Geometry: final body of the model. Coordinates: model frame, mm. Face numbers are marked on the shaded views. A direction names the side the tool comes from. Coordinates: 2 decimals unless noted, no trailing zeros. Loops run counter-clockwise (first coordinate to the right, second up) from the corner with the lowest first, then second, coordinate; pieces in that order, holes last. Notation, with made-up numbers: (-40, 10.5) -> (5, 10.5) arc R28 cw to (5, 45.5) -> close; hole circle Ø8 at (50, -9.75). An arc over 180 degrees is marked (long way). One line per item, written item: value. Start each with the question number.
Item 1: Mould query, pull axis Y, two halves, no side actions, for the marked faces 1, 2 and 3. Classes: +Y half, -Y half, draft (parallel to the pull), parting line (faces both ways), or undercut.
Item 2: Section query C-C on x = 36. Return loops of the section in (y, z) (3 decimals), then the cut area to 3 significant figures.
Item 3: Set-up query: the marked faces 4, 5, 6, 7 and 8. Return all of +Z, -Z, +X, -X, +Y, -Y with unobstructed straight access to the full face (end or side cutting, diameter ignored); none if empty.
Item 4: Section query A-A on y = 12.7. Return loops of the section in (x, z) (3 decimals), then the cut area to 3 significant figures.
Item 5: Contact query for flat-ended pins moving along their axis: pin 1 Ø4 at (x, y) = (38.5, -47.5) entering from -Z; pin 2 Ø3 at (y, z) = (-28.5, 12.5) entering from -X; pin 3 Ø3.5 at (y, z) = (-12.7, 0) entering from -X; pin 4 Ø10 at (y, z) = (-49.5, 4) entering from +X. Output: stop coordinate, or through.
Item 6: Section query B-B on y = -15. Return loops of the section in (x, z) (3 decimals), then the cut area to 3 significant figures.
Item 7: Ray query, probe 1 along X at (y, z) = (-3.5, 10); probe 2 along Y at (x, z) = (-4, 0) (3 decimals); probe 3 along Y at (x, z) = (32.1, 0) (3 decimals). Return the intervals inside material, ascending. Write a range as from..to.
Item 8: Section query D-D on x = 21.5. Return loops of the section in (y, z) (3 decimals).
from build123d import *

# Parameters (mm, degrees)
SKETCH1_R               = 15.875
SKETCH1_R_2             = 9.5
BOSS_EXTRUDE1_DEPTH     = 6
BOSS_EXTRUDE2_START     = 13.050000062
SKETCH2_R               = 15.875
SKETCH2_R_2             = 9.5
SKETCH2_R_3             = 7.62
BOSS_EXTRUDE2_DEPTH     = 13.050000062
BOSS_EXTRUDE3_START     = -19.050000062
BOSS_EXTRUDE3_DEPTH     = 19.050000062
BOSS_EXTRUDE4_START     = 21.59
BOSS_EXTRUDE4_DEPTH     = 19.050000062
BOSS_EXTRUDE5_REACH     = 71.404
CUT_EXTRUDE1_START      = -31.75
CUT_EXTRUDE1_DEPTH      = 31.75
SKETCH9_W               = 19.05
SKETCH9_H               = 19.05
BOSS_EXTRUDE8_DEPTH     = 31.75
CHAMFER1_SIZE           = 5.08
SKETCH6_R               = 7.62
SKETCH6_R_2             = 5.25
BOSS_EXTRUDE6_DEPTH     = 13.050000062
SKETCH7_R               = 1.5
CUT_EXTRUDE2_DEPTH      = 12.7
CUT_EXTRUDE3_REACH      = 90.091
CUT_EXTRUDE3_END_RADIUS = 5.25
SKETCH8_R               = 1.5
CUT_EXTRUDE4_REACH      = 86.149
SKETCH10_R              = 5.5
SKETCH10_R_2            = 5.25


# Read off the part's stored shape, not the designer's step: Cut-Extrude1
with BuildPart() as part:
    # Sketch1 → Boss-Extrude1 (new body)
    with BuildSketch(Plane(origin=(0, 0, 0), x_dir=(0, 0, -1), z_dir=(1, 0, 0))):
        Circle(SKETCH1_R)
        Circle(SKETCH1_R_2, mode=Mode.SUBTRACT)
    extrude(amount=BOSS_EXTRUDE1_DEPTH)

    # Sketch2 → Boss-Extrude2 (add)
    # profile 1 of 2: a face of its own
    with BuildSketch(Plane.ZY.offset(BOSS_EXTRUDE2_START)):
        Circle(SKETCH2_R)
        with Locations(Location((0, 0, 0), (0, 0, 180))):
            Circle(SKETCH2_R_2, mode=Mode.SUBTRACT)
    # profile 2 of 2: a face of its own
    with BuildSketch(Plane.ZY.offset(BOSS_EXTRUDE2_START)):
        with Locations(Location((0, 0, 0), (0, 0, 180))):
            Circle(SKETCH2_R_2)
        with Locations(Location((0, 0, 0), (0, 0, 180))):
            Circle(SKETCH2_R_3, mode=Mode.SUBTRACT)
    extrude(amount=-BOSS_EXTRUDE2_DEPTH)


with BuildPart() as body_2:
    # Mirror2: mirrored copy
    add(part.part.mirror(Plane(origin=(16.795, 0, 0), x_dir=(0, 0, 1), z_dir=(1, 0, 0))))

    # Sketch3<3> → Boss-Extrude4 (add)
    with BuildSketch(Plane(origin=(6, 0, 0), x_dir=(0, 0, -1), z_dir=(1, 0, 0)).offset(BOSS_EXTRUDE4_START)):
        with BuildLine():
            ThreePointArc((15.875, 0), (0, -15.875), (-15.875, 0))
            Line((-15.875, 0), (-15.875, -38.1))
            ThreePointArc((-15.875, -38.1), (0, -53.975), (15.875, -38.1))
            Line((15.875, -38.1), (15.875, 0))
        make_face()
    extrude(amount=BOSS_EXTRUDE4_DEPTH)

    # Sketch4 → Boss-Extrude5 (add, up to next)
    with BuildSketch(Plane(origin=(6, 0, 0), x_dir=(0, 0, -1), z_dir=(1, 0, 0)), mode=Mode.PRIVATE) as boss_extrude5_sk1:
        with BuildLine():
            Line((15.875, -25.4), (-15.875, -25.4))
            Line((-15.875, -25.4), (-15.875, -38.1))
            ThreePointArc((-15.875, -38.1), (0, -53.975), (15.875, -38.1))
            Line((15.875, -38.1), (15.875, -25.4))
        make_face()
    boss_extrude5_tool1 = extrude(boss_extrude5_sk1.sketch, amount=BOSS_EXTRUDE5_REACH, mode=Mode.PRIVATE) - body_2.part


with BuildPart() as part_1:
    add(part.part)

    # Sketch3 → Boss-Extrude3 (add)
    with BuildSketch(Plane(origin=(6, 0, 0), x_dir=(0, 0, -1), z_dir=(1, 0, 0)).offset(BOSS_EXTRUDE3_START)):
        with BuildLine():
            ThreePointArc((15.875, 0), (0, -15.875), (-15.875, 0))
            Line((-15.875, 0), (-15.875, -38.1))
            ThreePointArc((-15.875, -38.1), (0, -53.975), (15.875, -38.1))
            Line((15.875, -38.1), (15.875, 0))
        make_face()
    extrude(amount=BOSS_EXTRUDE3_DEPTH)


with BuildPart() as body_2_1:
    add(body_2.part)

    add(part_1.part)  # Boss-Extrude5 merges part
    add(boss_extrude5_tool1.solids().sort_by_distance((6, -38.23351, 0))[0])

    # Cut-Extrude1 outline → Cut-Extrude1 (cut)
    with BuildSketch(Plane.XY.offset(15.875).offset(CUT_EXTRUDE1_START)):
        with BuildLine():
            Line((-13.050000062, -15.875), (-13.050000062, -53.975))
            Line((-13.050000062, -53.975), (7.27, -53.975))
            ThreePointArc((7.27, -53.975), (-7.652500044, -37.465000015), (-13.050000062, -15.875))
        make_face()
        with BuildLine():
            ThreePointArc((46.640000062, -15.875), (41.242500044, -37.465000015), (26.32, -53.975))
            Line((26.32, -53.975), (46.640000062, -53.975))
            Line((46.640000062, -53.975), (46.640000062, -15.875))
        make_face()
    extrude(amount=CUT_EXTRUDE1_DEPTH, mode=Mode.SUBTRACT)

    # Sketch9 → Boss-Extrude8 (add)
    with BuildSketch(Plane(origin=(0, -25.4, 0), x_dir=(1, 0, 0), z_dir=(0, 1, 0))):
        with Locations((16.571454424, 0)):
            Rectangle(SKETCH9_W, SKETCH9_H)
    extrude(amount=-BOSS_EXTRUDE8_DEPTH)

    # Chamfer1
    chamfer1_edges = [body_2_1.edges().sort_by_distance(p)[0] for p in [
        (6, -25.4, 0),
        (27.59, -25.4, 0),
    ]]
    chamfer(chamfer1_edges, length=CHAMFER1_SIZE)

    # Sketch6 → Boss-Extrude6 (add)
    with BuildSketch(Plane(origin=(46.640000062, 0, 0), x_dir=(0, 0, -1), z_dir=(1, 0, 0))):
        Circle(SKETCH6_R)
        Circle(SKETCH6_R_2, mode=Mode.SUBTRACT)
    extrude(amount=-BOSS_EXTRUDE6_DEPTH)

    # Sketch7 → Cut-Extrude2 (cut)
    with BuildSketch(Plane.ZY.offset(13.050000062)):
        with Locations((0, 12.7)):
            Circle(SKETCH7_R)
        with Locations((0, -12.7)):
            Circle(SKETCH7_R)
    extrude(amount=-CUT_EXTRUDE2_DEPTH, mode=Mode.SUBTRACT)

    # Cut-Extrude3: up to this cylinder (the profile starts outside it)
    cut_extrude3_end = Plane(origin=(39.02, 0, 0), z_dir=(1, 0, 0)) * Cylinder(CUT_EXTRUDE3_END_RADIUS, 191.682, mode=Mode.PRIVATE)
    # Sketch8 → Cut-Extrude3 (cut, up to the surface)
    with BuildSketch(Plane(origin=(0, 15.875, 0), x_dir=(1, 0, 0), z_dir=(0, 1, 0)), mode=Mode.PRIVATE) as cut_extrude3_sk1:
        with Locations(Location((39.020000062, 0, 0), (0, 0, 270))):
            Circle(SKETCH8_R)
    cut_extrude3_tool1 = extrude(cut_extrude3_sk1.sketch, amount=-CUT_EXTRUDE3_REACH, mode=Mode.PRIVATE) - cut_extrude3_end
    add(cut_extrude3_tool1.solids().sort_by_distance((39.02, 15.875, 0))[0], mode=Mode.SUBTRACT)

    # Cut-Extrude4: up to this face of the body (flat: up to its plane)
    cut_extrude4_end = Plane(body_2_1.part.faces().sort_by_distance((33.59, 0, 9.231299423))[0])
    # Sketch10 → Cut-Extrude4 (cut, up to the picked face)
    with BuildSketch(Plane(origin=(46.640000062, 0, 0), x_dir=(0, 0, -1), z_dir=(1, 0, 0)), mode=Mode.PRIVATE) as cut_extrude4_sk1:
        Circle(SKETCH10_R)
        Circle(SKETCH10_R_2, mode=Mode.SUBTRACT)
    cut_extrude4_tool1 = split(extrude(cut_extrude4_sk1.sketch, amount=-CUT_EXTRUDE4_REACH, mode=Mode.PRIVATE), bisect_by=cut_extrude4_end, keep=Keep.BOTH, mode=Mode.PRIVATE)
    # Sketch10 → Cut-Extrude4 (cut, up to the picked face)
    with BuildSketch(Plane(origin=(46.640000062, 0, 0), x_dir=(0, 0, -1), z_dir=(1, 0, 0)), mode=Mode.PRIVATE) as cut_extrude4_sk2:
        Circle(SKETCH10_R_2)
    cut_extrude4_tool2 = split(extrude(cut_extrude4_sk2.sketch, amount=-CUT_EXTRUDE4_REACH, mode=Mode.PRIVATE), bisect_by=cut_extrude4_end, keep=Keep.BOTH, mode=Mode.PRIVATE)
    add(cut_extrude4_tool1.solids().sort_by(Axis((46.64, 0, 5.344437), (-1, 0, 0)))[0], mode=Mode.SUBTRACT)
    add(cut_extrude4_tool2.solids().sort_by(Axis((46.64, 0, 0), (-1, 0, 0)))[0], mode=Mode.SUBTRACT)


solid = body_2_1.part
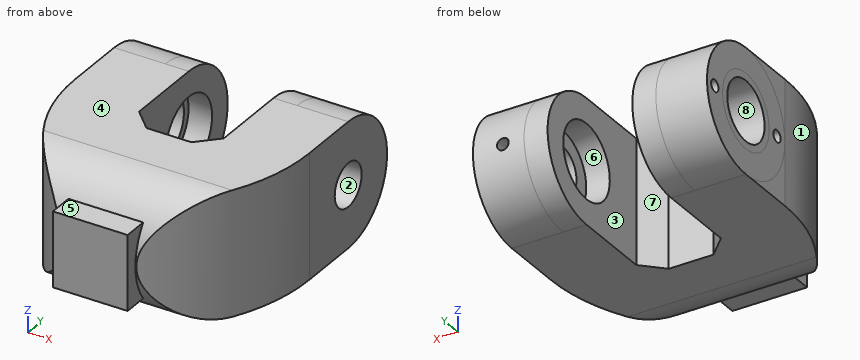
Reply:
1. face 1: -Y half
1. face 2: undercut
1. face 3: draft
2. outline: (-45.253, -14.172) arc R15.875 ccw to (-38.1, -15.875) -> (0, -15.875) arc R15.875 ccw to (0, 15.875) -> (-38.1, 15.875) arc R15.875 ccw to (-45.253, 14.172) -> close; hole circle Ø11 at (0, 0)
2. area: 1,730 mm²
3. face 4: +Z, +X, -X, +Y, -Y
3. face 5: +Z, +X, -X, -Y
3. face 6: none
3. face 7: +Z, -Z, +Y
3. face 8: -X
4. outline: (-13.05, -9.525) -> (6, -9.525) -> (6, 9.525) -> (-13.05, 9.525) -> (-13.05, 1.5) -> (-0.35, 1.5) -> (-0.35, -1.5) -> (-13.05, -1.5) -> close; (27.59, -9.525) -> (46.64, -9.525) -> (46.64, 9.525) -> (27.59, 9.525) -> close; hole circle Ø3 at (39.02, 0)
4. area: 681 mm²
5. pin 1: passes through
5. pin 2: stops at x = -11.68
5. pin 3: stops at x = -13.05
5. pin 4: stops at x = 36.61
6. outline: (-13.05, -15.875) -> (6, -15.875) -> (6, 15.875) -> (-13.05, 15.875) -> close; (27.59, -15.875) -> (46.64, -15.875) -> (46.64, 15.875) -> (27.59, 15.875) -> close
6. area: 1,210 mm²
7. probe 1: x = -13.05..6, 27.59..46.64
7. probe 2: y = -43.234..-14.2, -11.2..-7.62, 7.62..11.2, 14.2..15.875
7. probe 3: y = -49.382..-9.5, 9.5..15.875
8. outline: (-57.15, -9.525) -> (-50.8, -9.525) arc R15.875 ccw to (-38.1, -15.875) -> (-25.4, -15.875) -> (-25.4, 15.875) -> (-38.1, 15.875) arc R15.875 ccw to (-50.8, 9.525) -> (-57.15, 9.525) -> close
